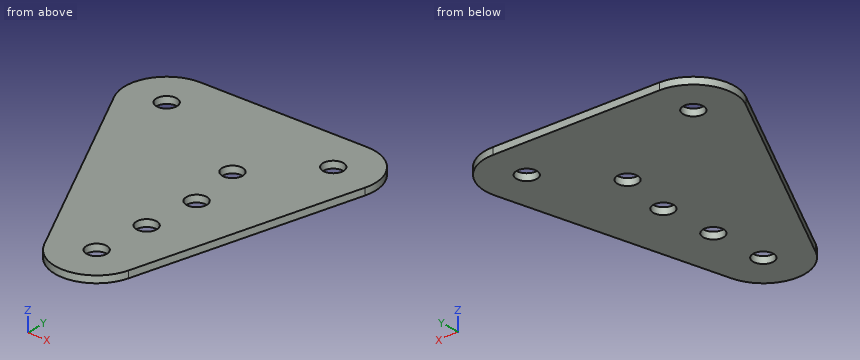
Autodesk Inventor part; units mm, degrees
ref_plane "YZ Plane" through (0, 0, 0) normal (1, 0, 0) x (0, 1, 0)
ref_plane "XZ Plane" through (0, 0, 0) normal (0, 1, 0) x (-1, 0, 0)
ref_plane "XY Plane" through (0, 0, 0) normal (0, 0, 1) x (1, 0, 0)
sketch "Sketch1" plane through (0, 0, 0) normal (0, 0, 1) x (1, 0, 0)
  circle A0 centre (-322.5487, -9.4748) radius 2.3368
  circle A1 centre (-321.4418, 3.1768) radius 2.3368
  circle A2 centre (-323.6556, -22.1265) radius 2.3368
  line L0 (-321.4418, 3.1768) -> (-321.0479, 7.6801) construction
  circle A3 centre (-367.8, 21.9203) radius 2.3114 construction
  line L1 (-378.0119, 9.2203) -> (-319.4881, 9.2203) construction
  circle A4 centre (-323.6556, -22.1265) radius 9.525
  circle A5 centre (-321.4418, 3.1768) radius 9.525
  circle A6 centre (-310.65, 28.2703) radius 2.3114 construction
  circle A7 centre (-323.35, 15.5703) radius 2.3114 construction
  circle A8 centre (-348.75, 28.2703) radius 9.525
  circle A9 centre (-310.65, 28.2703) radius 9.525
  line L2 (-332.182, -26.3721) -> (-357.2764, 24.0247)
  line L3 (-312.0866, 0.8208) -> (-311.9531, 2.3467)
  line L4 (-312.6917, -0.5863) -> (-312.0866, 0.8208)
  line L5 (-310.65, 37.7953) -> (-348.75, 37.7953)
  line L6 (-346.4386, 30.0737) -> (-346.4386, 26.4669) construction
  circle A10 centre (-348.75, 28.2703) radius 2.3114 construction
  circle A11 centre (-348.75, 28.2703) radius 2.3368
  circle A12 centre (-310.65, 28.2703) radius 2.3368
  circle A13 centre (-323.35, 15.5703) radius 2.3368
  circle A14 centre (-321.4418, 3.1768) radius 1.5848 construction
  circle A15 centre (-321.4418, 3.1768) radius 1.5848 construction
  line L7 (-314.4328, -24.5066) -> (-301.4272, 25.8902)
  point P0 (0, 0)
  point P1 (-319.4881, 34.6203)
  point P2 (-314.4552, -24.5918)
  point P3 (-301.8999, 24.5072)
  point P4 (-312.4196, 0.0464)
  dimension "d0" = 4.6736
  dimension "d1" = 4.6736
  dimension "d2" = 4.6736
  dimension "d5" = 0
  dimension "d6" = 0
  dimension "d8" = 85
  dimension "d9" = 19.05
  dimension "d10" = 19.05
  dimension "d11" = 19.05
  dimension "d12" = 19.05
  dimension "d13" = 0
  dimension "d14" = 0
  dimension "d15" = 4.6736
  dimension "d16" = 4.6736
  dimension "d17" = 4.6736
  dimension "d20" = 0
  dimension "d22" = 12.7
  dimension "d23" = 12.7
  dimension "d24" = 0
extrude "Extrusion2" add sketch "Sketch1" along normal blind 1.5875 contours A4 | A4 L2 A8 L5 A9 L7 | A8 | A9 | A5
sketch "Sketch2" plane through (0, 0, 1.5875) normal (0, 0, 1) x (1, 0, 0)
  arc A0 (-312.6917, -0.5863) -> (-311.9531, 2.3467) centre (-321.4418, 3.1768) ccw
  line L0 (-312.0866, 0.8208) -> (-312.6917, -0.5863)
  line L1 (-311.9531, 2.3467) -> (-312.0866, 0.8208)
  arc A1 (-301.4272, 25.8902) -> (-310.65, 37.7953) centre (-310.65, 28.2703) ccw
  line L2 (-310.65, 37.7953) -> (-348.75, 37.7953)
  arc A2 (-348.75, 37.7953) -> (-357.2764, 24.0247) centre (-348.75, 28.2703) ccw
  line L3 (-357.2764, 24.0247) -> (-332.182, -26.3721)
  arc A3 (-332.182, -26.3721) -> (-314.4328, -24.5066) centre (-323.6556, -22.1265) ccw
  line L4 (-314.4328, -24.5066) -> (-301.4272, 25.8902)
  circle A4 centre (-321.4418, 3.1768) radius 2.3368
  circle A5 centre (-323.6556, -22.1265) radius 2.3368
  circle A6 centre (-348.75, 28.2703) radius 2.3368
  circle A7 centre (-310.65, 28.2703) radius 2.3368
  circle A8 centre (-323.35, 15.5703) radius 2.3368
  circle A9 centre (-322.5487, -9.4748) radius 2.3368
  line L5 (-312.0866, 0.8208) -> (-312.6917, -0.5863)
  arc A10 (-312.6917, -0.5863) -> (-311.9531, 2.3467) centre (-321.4418, 3.1768) ccw
  line L6 (-311.9531, 2.3467) -> (-312.0866, 0.8208)
  point P0 (0, 0)
sheet face with bend "Face1" sketch "Sketch2" thickness 1.5875 toward (0, 0, -1) bend radius 1.5875 contours A0 L1 L0
bend "Bend1"
equation "\"d27\" = Thickness"
equation "\"d28\" = BendRadius"
equation "\"d29\" = BendReliefWidth"
equation "\"d31\" = MinimumRemnant"
equation "\"d30\" = BendReliefDepth"
equation "\"d32\" = TransitionRadius"
equation "\"BendRadius\" = Thickness"
equation "\"BendReliefWidth\" = Thickness"
equation "\"BendReliefDepth\" = 0.5 * Thickness"
equation "\"CornerReliefSize\" = 4 * Thickness"
equation "\"MinimumRemnant\" = 2 * Thickness"
equation "\"TransitionRadius\" = BendRadius"
equation "\"JacobiRadiusSize\" = BendRadius"
equation "\"GapSize\" = Thickness"
properties part number "motormount"
Geometry: final body of the model. Coordinates: model frame, mm. Give positions to 0.01 mm unless a question says otherwise; leave off trailing zeros. Loops run counter-clockwise (first coordinate to the right, second up) from the corner with the lowest first, then second, coordinate; pieces in that order, holes last. Notation, with made-up numbers: (74, 7.25) - (102, 7.25) arc R26 ccw to (102, 31.25) - close; hole circle Ø2 at (77.25, -3). An arc over 180 degrees is marked (long way). Answer as CSV lines item,"result". Start each with the question number.
1. Section A-A, the plane z = 1. Give the number of separate pieces and of enclosed holes in the cut face, plus the area to 3 significant figures.
2. Pin query (flat end, axial travel): P1, Ø4, axis at x = -322.55, y = -9.47, coming from the -Z side. Return the tip coordinate at first contact, or that it passes through.
3. Section B-B, the plane y = -17.5. Return loops of the section in (x, z), plus the area to 3 significant figures.
4. Ray query, L1, parallel to Y at x = -322.5, z = 0.65; L2, parallel to X at y = 16.5, z = 1.15; L3, parallel to Y at x = -320.5, z = 0.85. Return the intervals inside material, ascending.
5. Section C-C, the plane y = -2. Return loops of the section in (x, z), plus the area to 3 significant figures.
Answers:
1,separate pieces,"1"
1,enclosed holes,"6"
1,area,"2,540 mm2"
2,P1,"passes through"
3,outline,"(-336.6, 0) - (-312.62, 0) - (-312.62, 1.59) - (-336.6, 1.59) - close"
3,area,"38.1 mm2"
4,L1,"y = -31.58 to -24.16, -20.1 to -11.81, -7.14 to 1.09, 5.26 to 13.39, 17.75 to 37.8"
4,L2,"x = -353.53 to -325.49, -321.21 to -303.85"
4,L3,"y = -31.11 to -10.6, -8.35 to 1.04, 5.32 to 37.8"
5,outline,"(-344.32, 0) - (-308.62, 0) - (-308.62, 1.59) - (-344.32, 1.59) - close"
5,area,"56.7 mm2"
